```python
from build123d import *

# Parameters (mm, degrees)
F0_W     = 2.8
F0_H     = 8
F1_DEPTH = 48.5
F2_R     = 3.99999
F3_R     = 1.5
F4_DEPTH = 5
F5_R     = 0.5


# Not quite as in the source:
# - a fillet or chamfer is up to 0.001 mm smaller than in the source, because OpenCascade refuses the exact size


with BuildPart() as f1:
    # F0 (on Top) → F1 (new body)
    with BuildSketch(Plane.XY):
        Rectangle(F0_W, F0_H)
    extrude(amount=F1_DEPTH)

    # F2 (radius 4 in the source; OpenCascade refuses exactly that, so slightly less here)
    f2_edges = [f1.edges().sort_by_distance(p)[0] for p in [
        (0, 4, 0),
        (0, -4, 0),
        (0, -4, 48.5),
        (0, 4, 48.5),
    ]]
    fillet(f2_edges, radius=F2_R)

    # F3 (on face) → F4 (cut)
    with BuildSketch(Plane(origin=(-1.4, 0, 0), x_dir=(0, -1, 0), z_dir=(-1, 0, 0))):
        with Locations((0, 4)):
            Circle(F3_R)
        with Locations((0, 44.5)):
            Circle(F3_R)
    extrude(amount=-F4_DEPTH, mode=Mode.SUBTRACT)

    # F5
    f5_edges = [f1.edges().sort_by_distance(p)[0] for p in [
        (-1.4, 4, 24.25),
        (1.4, 4, 24.25),
    ]]
    fillet(f5_edges, radius=F5_R)


solid = f1.part
```
Model file for the job. Use its own axes, mm. Coordinates: 2 decimals unless noted, no trailing zeros. Answer as a JSON object with one key per item and string values. Group by question number.
(1) Probe line 1 along Z through (x, y) = (0.65, 0); line 2 along Z through (x, y) = (-0.05, 0.5); line 3 along Y through (x, z) = (-0.6, 2). List the from-to ranges inside material, lowest first.
(2) Flat gauge pin, fed straight in: pin 1 (1.5 mm diameter, centred on x = 0.5, y = 2.5, fed in from +Z). Where does the tip first touch, or does it go through?
(3) Two-plate mould, pull along Z, no slides. Class faces 1 (the face through (0.013, 2.859, 47.297)), 2 (the face through (-0.02, -0.806, 5.265)), 3 (the face through (1.4, 0, 24)): released by +Z, released by -Z, zero draft, split by the parting line, or undercut.
(4) Cut at A-A (x = 0). State how many separate pieces and enclosed holes the cut face has, then the cut area to 3 significant figures.
Geometry says:
{
 "1": {"line 1": "z = 0 to 2.5, 5.5 to 43, 46 to 48.5", "line 2": "z = 0.03 to 2.59, 5.41 to 43.09, 45.91 to 48.47", "line 3": "y = -3.46 to 3.46"},
 "2": {"pin 1": "stops at z = 48.1"},
 "3": {"face 1": "released by +Z", "face 2": "undercut", "face 3": "zero draft"},
 "4": {"separate pieces": "1", "enclosed holes": "2", "area": "360 mm^2"}
}
